```python
from build123d import *

# Parameters (mm, degrees)
BOSS_EXTRUDE4_DEPTH = 12.7
FILLET5_R           = 31.75
FILLET6_R           = 25.4
BOSS_EXTRUDE5_START = 63.5
BOSS_EXTRUDE5_DEPTH = 12.7
SKETCH20_R          = 6.35
CUT_EXTRUDE6_DEPTH  = 112.014
FILLET7_R           = 12.7
CHAMFER2_SIZE       = 2.54
BOSS_EXTRUDE7_START = 50.8
SKETCH22_R          = 6.35
BOSS_EXTRUDE7_DEPTH = 12.7
SKETCH23_R          = 3.175


with BuildPart() as part:
    # Sketch2 → Revolve1 (revolve)
    with BuildSketch(Plane.XY):
        with BuildLine():
            Line((0, 31.75), (0, 0))
            Line((0, 0), (0, -31.75))
            ThreePointArc((0, -31.75), (31.75, 0), (0, 31.75))
        make_face()
    revolve(axis=Axis((0, 31.75, 0), (0, -1, 0)))

    # Sketch15 → Boss-Extrude4 (add, symmetric)
    with BuildSketch(Plane.XY):
        Polygon((0, 0), (0, 6.35), (-53.34, 6.35), (-121.3358, 63.5), (-190.5, 63.5), (-190.5, 50.8), (-125.964099177, 50.8), (-57.968299177, -6.35), (-10.998522628, -6.35), (0, -6.35), align=None)
    extrude(amount=BOSS_EXTRUDE4_DEPTH, both=True)

    # Fillet5
    fillet5_edges = [part.edges().sort_by_distance(p)[0] for p in [
        (-53.34, 6.35, 0),
        (-121.3358, 63.5, 0),
    ]]
    fillet(fillet5_edges, radius=FILLET5_R)

    # Fillet6
    fillet6_edges = [part.edges().sort_by_distance(p)[0] for p in [
        (-125.964099177, 50.8, 0),
        (-57.968299177, -6.35, 0),
    ]]
    fillet(fillet6_edges, radius=FILLET6_R)

    # Sketch19 → Boss-Extrude5 (add)
    with BuildSketch(Plane(origin=(0, 0, 0), x_dir=(1, 0, 0), z_dir=(0, 1, 0)).offset(BOSS_EXTRUDE5_START)):
        Polygon((-134.630325886, 0), (-164.459837057, 41.056799873), (-212.725, 25.374497791), (-212.725, -25.374497791), (-164.459837057, -41.056799873), align=None)
    extrude(amount=-BOSS_EXTRUDE5_DEPTH)

    # Sketch20 → Cut-Extrude6 (cut)
    with BuildSketch(Plane(origin=(0, 0, 0), x_dir=(1, 0, 0), z_dir=(0, 1, 0))):
        with Locations(Location((-177.8, 0, 0), (0, 0, 90))):
            Circle(SKETCH20_R)
    extrude(amount=CUT_EXTRUDE6_DEPTH, mode=Mode.SUBTRACT)

    # Fillet7
    fillet7_edges = [part.edges().sort_by_distance(p)[0] for p in [
        (-164.459837057, 57.15, -41.056799873),
        (-143.857415991, 57.15, 12.7),
        (-164.459837057, 57.15, 41.056799873),
        (-212.725, 57.15, 25.374497791),
        (-212.725, 57.15, -25.374497791),
        (-143.857415991, 57.15, -12.7),
    ]]
    fillet(fillet7_edges, radius=FILLET7_R)

    # Chamfer2
    chamfer2_edges = [part.edges().sort_by_distance(p)[0] for p in [
        (-153.348624091, 63.5, 25.763527232),
        (-188.592418529, 63.5, -33.215648832),
        (-212.725, 63.5, 0),
        (-188.592418529, 63.5, 33.215648832),
        (-165.386289571, 63.5, 38.205472221),
        (-210.299515829, 63.5, 23.612280389),
        (-210.299515829, 63.5, -23.612280389),
        (-165.386289571, 63.5, -38.205472221),
        (-188.592418529, 50.8, -33.215648832),
        (-136.303570156, 50.8, 12.7),
        (-153.348624091, 50.8, 25.763527232),
        (-188.592418529, 50.8, 33.215648832),
        (-212.725, 50.8, 0),
        (-165.386289571, 50.8, 38.205472221),
        (-210.299515829, 50.8, 23.612280389),
        (-210.299515829, 50.8, -23.612280389),
        (-165.386289571, 50.8, -38.205472221),
        (-35.083657686, 6.35, -12.7),
        (-143.15212213, 63.5, -14.084217143),
        (-143.15212213, 50.8, -14.084217143),
        (-143.15212213, 63.5, 14.084217143),
        (-143.15212213, 50.8, 14.084217143),
        (-35.083657686, 6.35, 12.7),
        (-135.146495362, 63.5, -12.7),
        (-135.146495362, 63.5, 12.7),
        (-87.3379, 34.925, -12.7),
        (-122.035219306, 61.580801426, -12.7),
        (-87.3379, 34.925, 12.7),
        (-122.035219306, 61.580801426, 12.7),
        (-52.640580694, 8.269198574, -12.7),
        (-52.640580694, 8.269198574, 12.7),
        (-91.966199177, 22.225, -12.7),
        (-91.966199177, 22.225, 12.7),
        (-38.554882069, -6.35, -12.7),
        (-38.554882069, -6.35, 12.7),
        (-57.408763732, -4.81464114, -12.7),
        (-57.408763732, -4.81464114, 12.7),
        (-126.523634621, 49.26464114, -12.7),
        (-126.523634621, 49.26464114, 12.7),
        (-136.303570156, 50.8, -12.7),
        (-153.348624091, 50.8, -25.763527232),
        (-153.348624091, 63.5, -25.763527232),
    ]]
    chamfer(chamfer2_edges, length=CHAMFER2_SIZE)

    # Sketch22 → Boss-Extrude7 (add)
    with BuildSketch(Plane(origin=(0, 0, 0), x_dir=(1, 0, 0), z_dir=(0, 1, 0)).offset(BOSS_EXTRUDE7_START)):
        with Locations(Location((-198.349031657, -14.929745408, 0), (0, 0, 180))):
            Circle(SKETCH22_R)
        with Locations(Location((-198.349031657, 14.929745408, 0), (0, 0, 180))):
            Circle(SKETCH22_R)
        with Locations(Location((-169.950968343, 24.156835514, 0), (0, 0, 180))):
            Circle(SKETCH22_R)
        with Locations(Location((-169.950968343, -24.156835514, 0), (0, 0, 180))):
            Circle(SKETCH22_R)
    extrude(amount=-BOSS_EXTRUDE7_DEPTH)

    # Sketch23 → Cut-Revolve12 (revolve, cut)
    with BuildSketch(Plane.XY):
        with Locations((-15.875, 27.49630657)):
            Circle(SKETCH23_R)
    revolve(axis=Axis((0, 0, 0), (0.5000000000000011, 0.866025403784438, 0)), mode=Mode.SUBTRACT)


solid = part.part
```
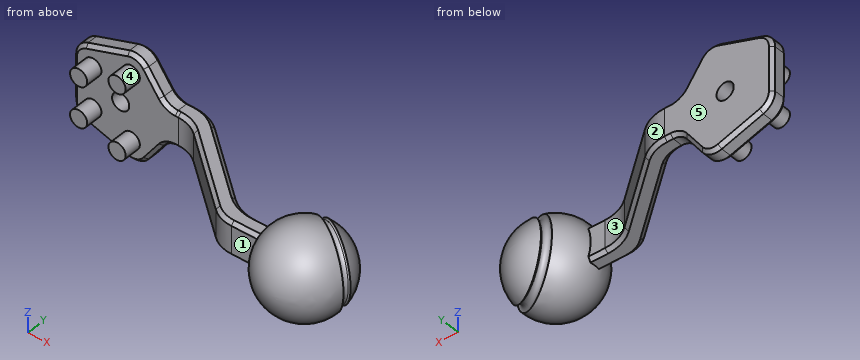
The model under review builds one solid part; all positions refer to its coordinate system, in mm. Face numbers are marked on the shaded views. A direction names the side the tool comes from. Round coordinates to 2 decimals unless told otherwise and drop trailing zeros. Order: outer loops, then holes, each group sorted by start corner. A loop starts at its lowest first (then second) coordinate and runs counter-clockwise, first axis right, second up.
Item 1: For pin 1 (4 mm diameter, centred on x = -199.5, z = -13, fed in from -Y); pin 2 (10 mm diameter, centred on x = -56, y = 4.5, fed in from +Z); pin 3 (14.5 mm diameter, centred on x = -177.8, z = 0, fed in from -Y); pin 4 (4 mm diameter, centred on x = -177.5, z = -5, fed in from +Y), all flat-tipped, find the tip position at first contact; note any pin that passes through.
Working result:
pin 1: stops at y = 38.1
pin 2: stops at z = 12.7
pin 3: stops at y = 50.8
pin 4: stops at y = 63.5
Item 2: Add section A-A, the plane z = 0. State the section outline as (x, y) points (3 decimals).
Working result:
outline: (-212.725, 53.34) - (-210.185, 50.8) - (-184.15, 50.8) - (-184.15, 63.5) - (-210.185, 63.5) - (-212.725, 60.96) - close; (-171.45, 50.8) - (-135.221, 50.8) arc R25.4 cw to (-118.878, 44.844) - (-65.054, -0.394) arc R25.4 ccw to (-48.712, -6.35) - (-31.109, -6.35) arc R31.75 ccw to (31.591, -3.171) arc R3.175 cw to (31.591, 3.171) arc R31.75 ccw to (-13.049, 28.944) arc R3.175 cw to (-18.542, 25.773) arc R31.75 ccw to (-31.109, 6.35) - (-41.769, 6.35) arc R31.75 cw to (-62.198, 13.795) - (-112.478, 56.055) arc R31.75 ccw to (-132.907, 63.5) - (-171.45, 63.5) - close
Item 3: Machinability: for the marked faces 4 and 5, which of the approach directions +Z, -Z, +X, -X, +Y, -Y give a long, thin tool a straight path to every point of the face, cutting with its end or side? Answer none if there is none.
Working result:
face 4: -Y
face 5: +Z, -Z, +X, -X, +Y
Item 4: To check wall thickness, follow probe 1 along X at (y, z) = (58.75, 0) (3 decimals); probe 2 along X at (y, z) = (57.5, 0) (3 decimals); probe 3 along Z at (x, y) = (-177, 59). State the ranges of each line that lie inside material, in increasing order.
Working result:
probe 1: x = -212.725 to -184.15, -171.45 to -116.201
probe 2: x = -212.725 to -184.15, -171.45 to -114.332
probe 3: z = -36.98 to -6.3, 6.3 to 36.98
Item 5: Draft analysis for pull direction X (two halves, no side actions). For the marked faces 1, 2 and 3, state which applies: released by +X, released by -X, zero draft, split by the parting line, or undercut.
Working result:
face 1: zero draft
face 2: released by +X
face 3: undercut
